from build123d import *

# Parameters (mm, degrees)
ESBO_O1_W                = 45.2
ESBO_O1_H                = 20.4
RESSALTO_EXTRUS_O1_DEPTH = 1
ESBO_O2_R                = 7.95
RESSALTO_EXTRUS_O2_DEPTH = 12.1
ESBO_O3_W                = 10
ESBO_O3_H                = 3.5
RESSALTO_EXTRUS_O3_DEPTH = 3.5
FILETE1_R                = 1.75
ESBO_O4_W                = 10
ESBO_O4_H                = 2.5
RESSALTO_EXTRUS_O4_DEPTH = 4
ESBO_O5_W                = 8
ESBO_O5_H                = 0.5
RESSALTO_EXTRUS_O5_DEPTH = 7.5
ESBO_O7_W                = 10
ESBO_O7_H                = 1.5
RESSALTO_EXTRUS_O6_DEPTH = 2.5


with BuildPart() as part:
    # Esboço1 → Ressalto-extrusão1 (new body)
    with BuildSketch(Plane.XY):
        with Locations((22.6, 10.2)):
            Rectangle(ESBO_O1_W, ESBO_O1_H)
    extrude(amount=RESSALTO_EXTRUS_O1_DEPTH)

    # Esboço2 → Ressalto-extrusão2 (add)
    with BuildSketch(Plane.XY.offset(1)):
        with Locations(Location((9.75, 10.2, 0), (0, 0, 180))):
            Circle(ESBO_O2_R)
        with Locations(Location((35.45, 10.2, 0), (0, 0, 180))):
            Circle(ESBO_O2_R)
    extrude(amount=RESSALTO_EXTRUS_O2_DEPTH)

    # Esboço3 → Ressalto-extrusão3 (add)
    with BuildSketch(Plane.XY.offset(1)):
        with Locations((22.6, 2.25)):
            Rectangle(ESBO_O3_W, ESBO_O3_H)
    extrude(amount=RESSALTO_EXTRUS_O3_DEPTH)

    # Filete1
    filete1_edges = [part.edges().sort_by_distance(p)[0] for p in [
        (27.6, 0.5, 2.75),
        (27.6, 4, 2.75),
        (17.6, 4, 2.75),
        (17.6, 0.5, 2.75),
    ]]
    fillet(filete1_edges, radius=FILETE1_R - 0.0001)  # a hair under: the kernel refuses the full size

    # Esboço4 → Ressalto-extrusão4 (add)
    with BuildSketch(Plane(origin=(0, 0, 0), x_dir=(-1, 0, 0), z_dir=(0, 0, -1))):
        with Locations((-22.6, 18.651439954)):
            Rectangle(ESBO_O4_W, ESBO_O4_H)
    extrude(amount=RESSALTO_EXTRUS_O4_DEPTH)

    # Esboço5 → Ressalto-extrusão5 (add)
    with BuildSketch(Plane(origin=(0, 19.901439954, 0), x_dir=(1, 0, 0), z_dir=(0, 1, 0))):
        with Locations((22.6, 3.75)):
            Rectangle(ESBO_O5_W, ESBO_O5_H)
    extrude(amount=RESSALTO_EXTRUS_O5_DEPTH)

    # Esboço7 → Ressalto-extrusão6 (add)
    with BuildSketch(Plane.XY.offset(1)):
        with Locations((22.6, 18.65)):
            Rectangle(ESBO_O7_W, ESBO_O7_H)
    extrude(amount=RESSALTO_EXTRUS_O6_DEPTH)


solid = part.part
Verification items for the finished model (mm, model axes). A direction names the side the tool comes from. Give positions to 0.01 mm unless a question says otherwise; leave off trailing zeros. Write each loop counter-clockwise with the first axis right and the second up, starting at its lowest first coordinate (ties: lowest second). Pieces come first, ordered by that corner, then holes. Notation, with made-up numbers: M 32.5,-26 L 69.5,-26 A19 cw 69.5,6 Z; hole C 79,88.5 d7. An arc over 180 degrees is marked long. Use CSV: the item, a comma, the result in double quotes.
1) Cross-section at B-B (y = 10.2). Enter the section's corners in (x, z), plus the area to 3 significant figures.
Final values:
outline,"M 0,0 L 45.2,0 L 45.2,1 L 43.4,1 L 43.4,13.1 L 27.5,13.1 L 27.5,1 L 17.7,1 L 17.7,13.1 L 1.8,13.1 L 1.8,1 L 0,1 Z"
area,"430 mm²"
2) Cross-section at D-D (x = 4). Enter the section's corners in (y, z), plus the area to 3 significant figures.
Final values:
outline,"M 0,0 L 20.4,0 L 20.4,1 L 15.69,1 L 15.69,13.1 L 4.71,13.1 L 4.71,1 L 0,1 Z"
area,"153 mm²"
3) Release check for a two-part mould opening along X. For faces 5 (the face through (23, 2, 4.5)), 6 (the face through (45.2, 10.1, 0.5)), 7 (the face through (36, 10, 13.1)) record: released by +X, released by -X, zero draft, split by the parting line, or undercut.
Final values:
face 5,"undercut"
face 6,"released by +X"
face 7,"zero draft"
4) Go/stop test with flat-tipped pins: pin 1 Ø2 at (y, z) = (18.5, -2) entering from -X; pin 2 Ø8 at (y, z) = (19, 10) entering from -X; pin 3 Ø3 at (x, z) = (7, 4.5) entering from +Y; pin 4 Ø1.5 at (x, y) = (30.5, 21.5) entering from -Z. Record where each tip stops, or that it passes through.
Final values:
pin 1,"x = 17.6"
pin 2,"x = 3.41"
pin 3,"y = 18.05"
pin 4,"through"
5) Cross-section at A-A (x = 35.45). Enter the section's corners in (y, z).
Final values:
outline,"M 0,0 L 20.4,0 L 20.4,1 L 18.15,1 L 18.15,13.1 L 2.25,13.1 L 2.25,1 L 0,1 Z"
6) Access from +Z, -Z, +X, -X, +Y, -Y to the whole of each face (thin tool, end or side, straight path). Record for faces 1 (the face through (23, 17.9, 2)), 2 (the face through (23, 17.401, -2)), 3 (the face through (17.6, 19, -2)), 4 (the face through (23, 19.4, 2)).
Final values:
face 1,"+Z"
face 2,"-Z, +X, -X, -Y"
face 3,"-Z, -X, +Y, -Y"
face 4,"+Z, +X, -X, +Y"
7) Material ranges on line 1 along Y through (x, z) = (20.5, 2); line 2 along Z through (x, y) = (27.5, 3.75); line 3 along X through (y, z) = (10.5, 10), recorded low to high.
Final values:
line 1,"0.5 to 4, 17.9 to 19.4"
line 2,"0 to 1"
line 3,"1.81 to 17.69, 27.51 to 43.39"
8) Cross-section at C-C (z = 9). Enter the section's corners in (x, y), plus the area to 3 significant figures.
Final values:
outline,"C 9.75,10.2 d15.9; C 35.45,10.2 d15.9"
area,"397 mm²"
